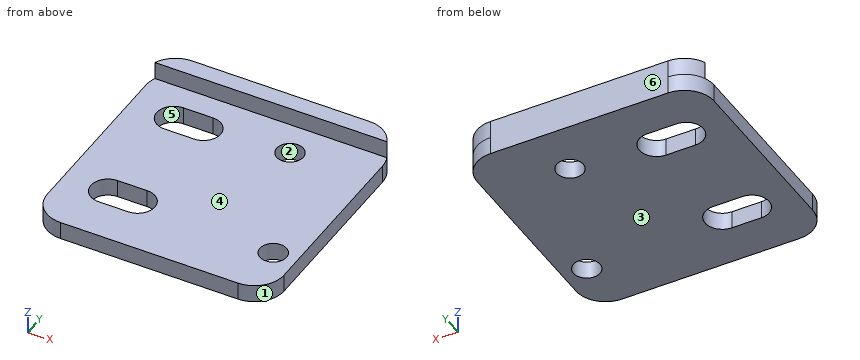
from build123d import *

# Parameters (mm, degrees)
SKETCH1_W                  = 40
SKETCH1_H                  = 40
BOSS_EXTRUDE1_DEPTH        = 3
F_4_5_4_5_DIAMETER_HOLE1_D = 4.5
M5_CLEARANCE_SLOT1_DEPTH   = 3
FILLET1_R                  = 5
BOSS_EXTRUDE2_START        = 3
BOSS_EXTRUDE2_DEPTH        = 3


# Read off the part's stored shape, not the designer's step: M5 Clearance Slot1
with BuildPart() as part:
    # Sketch1 → Boss-Extrude1 (new body)
    with BuildSketch(Plane.XY):
        with Locations((20, 20)):
            Rectangle(SKETCH1_W, SKETCH1_H)
    extrude(amount=BOSS_EXTRUDE1_DEPTH)

    # Ø4.5 (4.5) Diameter Hole1 (through all)
    with Locations(Plane.XY.offset(3)):
        with Locations((26.5, 31.1), (36, 8.9)):
            Hole(F_4_5_4_5_DIAMETER_HOLE1_D / 2)

    # M5 Clearance Slot1 outline → M5 Clearance Slot1 (cut)
    with BuildSketch(Plane.XY):
        with BuildLine():
            Line((7.5, 7.1), (12.5, 7.1))
            ThreePointArc((12.5, 7.1), (15.4, 10), (12.5, 12.9))
            Line((12.5, 12.9), (7.5, 12.9))
            ThreePointArc((7.5, 12.9), (4.6, 10), (7.5, 7.1))
        make_face()
        with BuildLine():
            Line((7.5, 27.1), (12.5, 27.1))
            ThreePointArc((12.5, 27.1), (15.4, 30), (12.5, 32.9))
            Line((12.5, 32.9), (7.5, 32.9))
            ThreePointArc((7.5, 32.9), (4.6, 30), (7.5, 27.1))
        make_face()
    extrude(amount=M5_CLEARANCE_SLOT1_DEPTH, mode=Mode.SUBTRACT)

    # Fillet1
    fillet1_edges = [part.edges().sort_by_distance(p)[0] for p in [
        (0, 40, 1.5),
        (40, 40, 1.5),
        (40, 0, 1.5),
        (0, 0, 1.5),
    ]]
    fillet(fillet1_edges, radius=FILLET1_R)

    # Sketch10 → Boss-Extrude2 (add)
    with BuildSketch(Plane.XY.offset(3).offset(BOSS_EXTRUDE2_START)):
        with BuildLine():
            Line((0.417424305, 37), (39.582575695, 37))
            ThreePointArc((39.582575695, 37), (37.738612788, 39.183300133), (35, 40))
            Line((35, 40), (5, 40))
            ThreePointArc((5, 40), (2.261387212, 39.183300133), (0.417424305, 37))
        make_face()
    extrude(amount=-BOSS_EXTRUDE2_DEPTH)


solid = part.part
Work out the finished part from the listing and answer in its coordinate system (mm). Face numbers are marked on the shaded views. A direction names the side the tool comes from. Give positions to 0.01 mm unless a question says otherwise; leave off trailing zeros. Order: outer loops, then holes, each group sorted by start corner. A loop starts at its lowest first (then second) coordinate and runs counter-clockwise, first axis right, second up. Notation, with made-up numbers: (69.5, 4.25) -> (99.5, 4.25) arc R17 ccw to (99.5, 15.25) -> close; hole circle Ø7 at (88.25, 68.25). An arc over 180 degrees is marked (long way). One line per item, written item: value.
Item 1: Flat-ended cylindrical pins translate along their axes: P1, Ø2.5, axis at x = 10.5, z = 4, coming from the -Y side; P2, Ø5, axis at x = 36, y = 8.9, coming from the +Z side; P3, Ø2, axis at y = 13, z = 5, coming from the -X side. Find the tip coordinate at first contact, or state that the pin passes through.
Answer sheet:
P1: y = 0
P2: z = 3
P3: through
Item 2: Find section D-D, the plane y = 31.1. Give the vertices of the cut face in (x, z).
Answer sheet:
outline: (0, 0) -> (4.82, 0) -> (4.82, 3) -> (0, 3) -> close; (15.18, 0) -> (24.25, 0) -> (24.25, 3) -> (15.18, 3) -> close; (28.75, 0) -> (40, 0) -> (40, 3) -> (28.75, 3) -> close
Item 3: Find section C-C, the plane x = 6. Give the vertices of the cut face in (y, z).
Answer sheet:
outline: (0, 0) -> (7.52, 0) -> (7.52, 3) -> (0, 3) -> close; (12.48, 0) -> (27.52, 0) -> (27.52, 3) -> (12.48, 3) -> close; (32.48, 0) -> (40, 0) -> (40, 6) -> (37, 6) -> (37, 3) -> (32.48, 3) -> close
Item 4: Find section B-B, the plane y = 10. Give the vertices of the cut face in (x, z).
Answer sheet:
outline: (0, 0) -> (4.6, 0) -> (4.6, 3) -> (0, 3) -> close; (15.4, 0) -> (34.04, 0) -> (34.04, 3) -> (15.4, 3) -> close; (37.96, 0) -> (40, 0) -> (40, 3) -> (37.96, 3) -> close
Item 5: Determine the mould class of the marked faces 1, 2 and 3 for opening direction Y: released by +Y, released by -Y, zero draft, split by the parting line, or undercut.
Answer sheet:
face 1: released by -Y
face 2: undercut
face 3: zero draft
Item 6: Find section A-A, the plane x = 26.5. Give the vertices of the cut face in (y, z), plus the area to 4 significant figures.
Answer sheet:
outline: (0, 0) -> (28.85, 0) -> (28.85, 3) -> (0, 3) -> close; (33.35, 0) -> (40, 0) -> (40, 6) -> (37, 6) -> (37, 3) -> (33.35, 3) -> close
area: 115.5 mm²
Item 7: Straight lines are drawn through the part: probe 1 along X at (y, z) = (8.5, 2.75); probe 2 along Y at (x, z) = (18, 5.65); probe 3 along Z at (x, y) = (20, 5). For each, find the intervals that lie inside material, in ascending order.
Answer sheet:
probe 1: 0 to 5.02, 14.98 to 33.79, 38.21 to 40
probe 2: 37 to 40
probe 3: 0 to 3
Item 8: A tool of negligible diameter and unlimited length cuts with its end or side. For the marked faces 4, 5 and 6, from which of +Z, -Z, +X, -X, +Y, -Y can it reach the whole face along a straight path? Write none if from no direction.
Answer sheet:
face 4: +Z, +X, -X, -Y
face 5: +Z, -Z
face 6: +Z, -Z, +X, -X, +Y
